The drawing under review shows one solid part. Ordinate dimensions are in mm from its lowest x, y, z. Coordinates: 2 decimals unless noted, no trailing zeros. Write each loop counter-clockwise with the first axis right and the second up, starting at its lowest first coordinate (ties: lowest second). Pieces come first, ordered by that corner, then holes.
1) Add section B-B, the plane y = 4.5. State the section outline as (x, z) points (3 decimals).
2) For P1, Ø10, axis at x = 3.5, z = 18.5, coming from the -Y side, flat-tipped, find the tip position at first contact; note if it passes through.
3) For line 1 (Y direction, x = 4.25, z = 74); line 2 (Z direction, x = 10, y = 2), list the stretches that pass through material, from the lowest coordinate up.
4) Add section C-C, the plane z = 49. State the section outline as (x, y) points, then the cut area to 3 significant figures.
5) Add section A-A, the plane x = 3. State the section outline as (y, z) points, then the cut area to 3 significant figures.
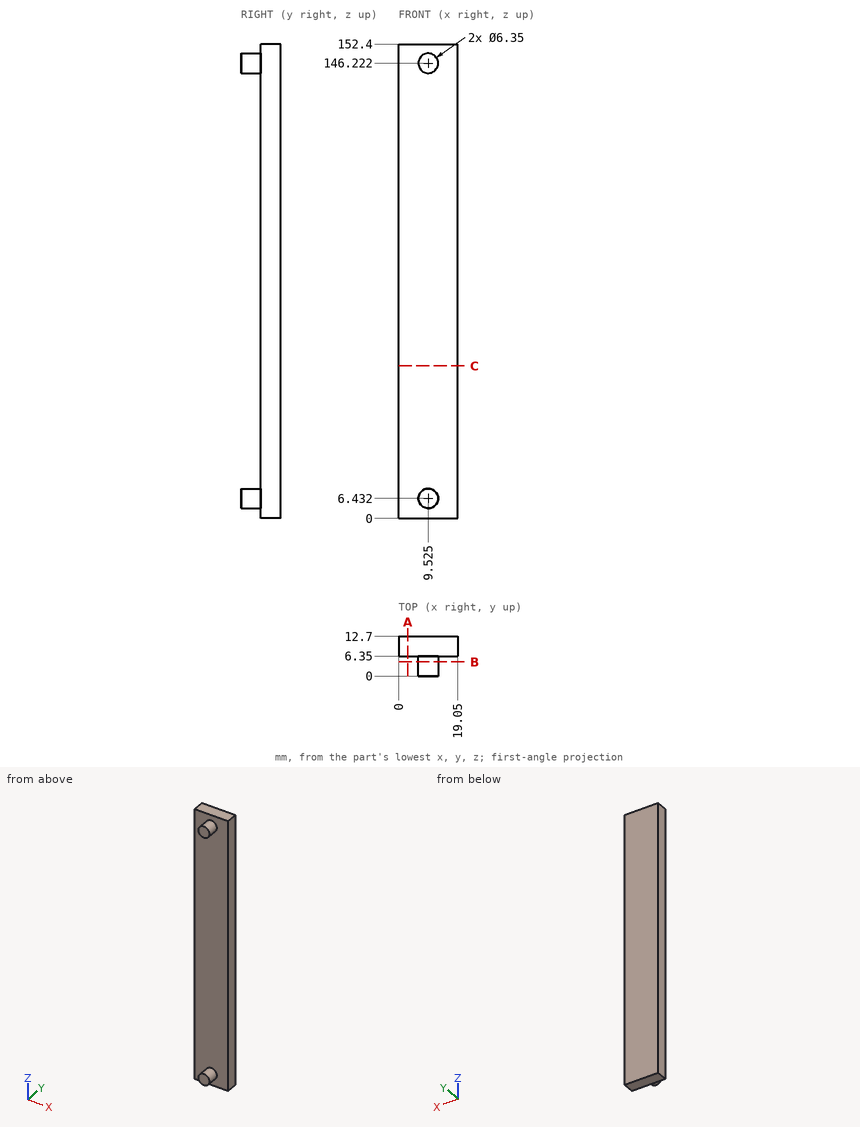
Geometry results:
1. outline: circle Ø6.35 at (9.525, 6.432); circle Ø6.35 at (9.525, 146.222)
2. P1: stops at y = 6.35
3. line 1: y = 6.35 to 12.7
3. line 2: z = 3.29 to 9.57, 143.08 to 149.36
4. outline: (0, 6.35) - (19.05, 6.35) - (19.05, 12.7) - (0, 12.7) - close
4. area: 121 mm2
5. outline: (6.35, 0) - (12.7, 0) - (12.7, 152.4) - (6.35, 152.4) - close
5. area: 968 mm2
